from build123d import *

# Parameters (mm, degrees)
SKETCH_1_W      = 75
SKETCH_1_H      = 70
SKETCH_1_R      = 1.5
SKETCH_1_W_2    = 52
SKETCH_1_H_2    = 55
SKETCH_1_W_3    = 90
SKETCH_1_W_4    = 30
EXTRUDE_1_DEPTH = 3
FILLET_1_R      = 10
FILLET_2_R      = 5
FILLET_3_R      = 10


with BuildPart() as part:
    # 草图1 → 凸台-拉伸1 (new body)
    # profile 1 of 3: a face of its own
    with BuildSketch(Plane(origin=(0, 0, 0), x_dir=(1, 0, 0), z_dir=(0, 1, 0))):
        Rectangle(SKETCH_1_W, SKETCH_1_H)
        with Locations(Location((-7.6, -28, 0), (0, 0, 270))):
            Circle(SKETCH_1_R, mode=Mode.SUBTRACT)
        with Locations(Location((-31, -20, 0), (0, 0, 270))):
            Circle(SKETCH_1_R, mode=Mode.SUBTRACT)
        with Locations(Location((-1, -30, 0), (0, 0, 270))):
            Circle(SKETCH_1_R, mode=Mode.SUBTRACT)
        with Locations(Location((31, -30, 0), (0, 0, 270))):
            Circle(SKETCH_1_R, mode=Mode.SUBTRACT)
        with Locations(Location((31, -20, 0), (0, 0, 270))):
            Circle(SKETCH_1_R, mode=Mode.SUBTRACT)
        with Locations((0, 5)):
            Rectangle(SKETCH_1_W_2, SKETCH_1_H_2, mode=Mode.SUBTRACT)
        with Locations(Location((-31, 20, 0), (0, 0, 270))):
            Circle(SKETCH_1_R, mode=Mode.SUBTRACT)
        with Locations(Location((31, 20, 0), (0, 0, 270))):
            Circle(SKETCH_1_R, mode=Mode.SUBTRACT)
    # profile 2 of 3: a face of its own
    with BuildSketch(Plane(origin=(0, 0, 0), x_dir=(1, 0, 0), z_dir=(0, 1, 0))):
        with Locations((-82.5, 0)):
            Rectangle(SKETCH_1_W_3, SKETCH_1_H)
        with Locations(Location((-122.4, -28, 0), (0, 0, 270))):
            Circle(SKETCH_1_R, mode=Mode.SUBTRACT)
        with Locations((-65, 5)):
            Rectangle(SKETCH_1_W_4, SKETCH_1_H_2, mode=Mode.SUBTRACT)
        with Locations((-103, 5)):
            Rectangle(SKETCH_1_W_4, SKETCH_1_H_2, mode=Mode.SUBTRACT)
    # profile 3 of 3: a face of its own
    with BuildSketch(Plane(origin=(0, 0, 0), x_dir=(1, 0, 0), z_dir=(0, 1, 0))):
        Polygon((-127.5, 35), (-37.5, 35), (37.5, 35), (37.5, 45), (-127.5, 45), align=None)
        with Locations(Location((-122.4, 38, 0), (0, 0, 270))):
            Circle(SKETCH_1_R, mode=Mode.SUBTRACT)
        with Locations(Location((-7.6, 38, 0), (0, 0, 270))):
            Circle(SKETCH_1_R, mode=Mode.SUBTRACT)
        with Locations(Location((-1, 40, 0), (0, 0, 270))):
            Circle(SKETCH_1_R, mode=Mode.SUBTRACT)
        with Locations(Location((31, 40, 0), (0, 0, 270))):
            Circle(SKETCH_1_R, mode=Mode.SUBTRACT)
    extrude(amount=EXTRUDE_1_DEPTH)

    # 圆角1
    fillet_1_edges = [part.edges().sort_by_distance(p)[0] for p in [
        (-88, 1.5, -32.5),
        (-118, 1.5, -32.5),
        (-118, 1.5, 22.5),
        (-88, 1.5, 22.5),
        (-50, 1.5, -32.5),
        (-80, 1.5, -32.5),
        (-80, 1.5, 22.5),
        (-50, 1.5, 22.5),
    ]]
    fillet(fillet_1_edges, radius=FILLET_1_R)

    # 圆角2
    fillet_2_edges = [part.edges().sort_by_distance(p)[0] for p in [
        (-127.5, 1.5, -45),
        (37.5, 1.5, -45),
        (37.5, 1.5, 35),
        (-127.5, 1.5, 35),
    ]]
    fillet(fillet_2_edges, radius=FILLET_2_R)

    # 圆角3
    fillet_3_edges = [part.edges().sort_by_distance(p)[0] for p in [
        (26, 1.5, -32.5),
        (-26, 1.5, -32.5),
        (-26, 1.5, 22.5),
        (26, 1.5, 22.5),
    ]]
    fillet(fillet_3_edges, radius=FILLET_3_R)


solid = part.part
Work out the finished part from the listing and answer in its coordinate system (mm). A direction names the side the tool comes from. Round coordinates to 2 decimals unless told otherwise and drop trailing zeros. Order: outer loops, then holes, each group sorted by start corner. A loop starts at its lowest first (then second) coordinate and runs counter-clockwise, first axis right, second up. Notation, with made-up numbers: M 85,30.25 L 126,30.25 A9 ccw 126,36.25 Z; hole C 2,62.5 d9. An arc over 180 degrees is marked long. One line per item, written item: value.
Q1. For faces 1 (the face through (-90.85, 1.52, 19.49)), 2 (the face through (36, 1.52, 33.57)), determine the directions among +Z, -Z, +X, -X, +Y, -Y from which every point of the face is accessible in a straight line to the end or side of a thin tool.
Derived:
face 1: +Y, -Y
face 2: +Z, +X, +Y, -Y
Q2. Determine the mould class of faces 3 (the face through (-6.59, 1.48, 26.89)), 4 (the face through (-46, 0, -6)), 5 (the face through (-44, 1, -45)) for opening direction Z: released by +Z, released by -Z, zero draft, split by the parting line, or undercut.
Derived:
face 3: undercut
face 4: zero draft
face 5: released by -Z
Q3. Straight lines are drawn through the part: line 1 (X direction, y = 1.25, z = -40); line 2 (X direction, y = 0.5, z = -13); line 3 (X direction, y = 2.2, z = 28). For each, find the intervals that lie inside material, in ascending order.
Derived:
line 1: -127.5 to -2.5, 0.5 to 29.5, 32.5 to 37.5
line 2: -127.5 to -118, -88 to -80, -50 to -26, 26 to 37.5
line 3: -127.5 to -123.9, -120.9 to -9.1, -6.1 to 37.5
Q4. Find section C-C on z = -3. Write down the section's boundary in (x, y).
Derived:
outline: M -127.5,0 L -118,0 L -118,3 L -127.5,3 Z; M -88,0 L -80,0 L -80,3 L -88,3 Z; M -50,0 L -26,0 L -26,3 L -50,3 Z; M 26,0 L 37.5,0 L 37.5,3 L 26,3 Z
Q5. Find section A-A on z = -20. Write down the section's boundary in (x, y).
Derived:
outline: M -127.5,0 L -118,0 L -118,3 L -127.5,3 Z; M -88,0 L -80,0 L -80,3 L -88,3 Z; M -50,0 L -32.5,0 L -32.5,3 L -50,3 Z; M -29.5,0 L -26,0 L -26,3 L -29.5,3 Z; M 26,0 L 29.5,0 L 29.5,3 L 26,3 Z; M 32.5,0 L 37.5,0 L 37.5,3 L 32.5,3 Z
Q6. Find section B-B on x = -1. Write down the section's boundary in (y, z), then the cut area to 3 significant figures.
Derived:
outline: M 0,-45 L 3,-45 L 3,-41.5 L 0,-41.5 Z; M 0,-38.5 L 3,-38.5 L 3,-32.5 L 0,-32.5 Z; M 0,22.5 L 3,22.5 L 3,28.5 L 0,28.5 Z; M 0,31.5 L 3,31.5 L 3,35 L 0,35 Z
area: 57.0 mm²
Q7. Find section D-D on y = 2.4. Give the number of separate pieces and of enclosed holes in the cut face, then the cut area to 3 significant figures.
Derived:
separate pieces: 1
enclosed holes: 15
area: 7,190 mm²
